The model under review builds one solid part; all positions refer to its coordinate system, in mm. Give positions to 0.01 mm unless a question says otherwise; leave off trailing zeros. Loops run counter-clockwise (first coordinate to the right, second up) from the corner with the lowest first, then second, coordinate; pieces in that order, holes last. Notation, with made-up numbers: M 74.5,6.5 L 124.5,6.5 A9 ccw 124.5,15.5 Z; hole C 85.5,21.25 d8. An arc over 180 degrees is marked long. Put each result on its own line as item: value. Start each with the question number.
from build123d import *

# Parameters (mm, degrees)
F0_W        = 71.12
F0_H        = 140.97
F1_DEPTH    = 15.24
F2_SIZE     = 10.16
F3_SIZE     = 5.08
F4_SIZE     = 5.08
F5_SIZE     = 2.54
F6_SIZE     = 2.54
F7_T1_DEPTH = 24.5183278918
F7_T3_DEPTH = 24.5183278918
F7_T5_DEPTH = 24.5183278918
F7_T7_DEPTH = 24.5183278918


# Not quite as in the source:
# - a fillet or chamfer that OpenCascade refuses, or shapes differently, is made with other operations: its cross-section is extruded or revolved along the edge and cut away or added


with BuildPart() as f1:
    # F0 (on Front) → F1 (new body)
    with BuildSketch(Plane.XZ):
        with Locations((-1.2450981867, 23.9183327848)):
            Rectangle(F0_W, F0_H)
    extrude(amount=F1_DEPTH)

    # F2
    f2_edges = [f1.edges().sort_by_distance(p)[0] for p in [
        (-1.245098, -15.24, 94.403333),
        (34.314902, -15.24, 23.918333),
        (-36.805098, -15.24, 23.918333),
        (-1.245098, -15.24, -46.566667),
    ]]
    chamfer(f2_edges, length=F2_SIZE)

    # F3
    f3_edges = [f1.edges().sort_by_distance(p)[0] for p in [
        (-26.645098, -15.24, 23.918333),
        (-1.245098, -15.24, -36.406667),
        (24.154902, -15.24, 23.918333),
        (-1.245098, -15.24, 84.243333),
    ]]
    chamfer(f3_edges, length=F3_SIZE)

    # F4
    f4_edges = [f1.edges().sort_by_distance(p)[0] for p in [
        (-1.245098, -15.24, 79.163333),
        (-1.245098, -15.24, -31.326667),
        (-21.565098, -15.24, 23.918333),
        (19.074902, -15.24, 23.918333),
    ]]
    chamfer(f4_edges, length=F4_SIZE)

    # F5
    f5_edges = [f1.edges().sort_by_distance(p)[0] for p in [
        (18.881556, -14.267984, 78.969987),
        (-21.371752, -14.267984, 78.969987),
        (-21.371752, -14.267984, -31.133321),
        (18.881556, -14.267984, -31.133321),
    ]]
    chamfer(f5_edges, length=F5_SIZE)

    # F6
    f6_edges = [f1.edges().sort_by_distance(p)[0] for p in [
        (-1.245098, -15.24, 74.083333),
        (-1.245098, -15.24, -26.246667),
    ]]
    chamfer(f6_edges, length=F6_SIZE)

    # F7: chamfer of 2.54 on 4 edges, made by hand

    # F7_s2 → F7_t1 (cut)
    with BuildSketch(Plane(origin=(29.0610725046, 29.0610725046, -29.0610725046), x_dir=(0.7071067812, -0.7071067812, 0), z_dir=(-0.5773502692, -0.5773502692, 0.5773502692))):
        Polygon((25.6566976907, -27.3564258793), (27.8564022163, -23.5464258793), (27.8564022163, -26.0864258793), align=None)
    extrude(amount=F7_T1_DEPTH, mode=Mode.SUBTRACT)

    # F7_s4 → F7_t3 (cut)
    with BuildSketch(Plane(origin=(45.0066276944, 45.0066276944, 45.0066276944), x_dir=(0.7071067812, -0.7071067812, 0), z_dir=(-0.5773502692, -0.5773502692, -0.5773502692))):
        Polygon((27.8564022163, 62.6048997598), (25.6566976907, 66.4148997598), (27.8564022163, 65.1448997598), align=None)
    extrude(amount=F7_T3_DEPTH, mode=Mode.SUBTRACT)

    # F7_s6 → F7_t5 (cut)
    with BuildSketch(Plane(origin=(-45.8366931523, 45.8366931523, 45.8366931523), x_dir=(0.7071067812, 0.7071067812, 0), z_dir=(0.5773502692, -0.5773502692, -0.5773502692))):
        Polygon((-29.6172369585, 61.5882813474), (-27.4175324329, 65.3982813474), (-29.6172369585, 64.1282813474), align=None)
    extrude(amount=F7_T5_DEPTH, mode=Mode.SUBTRACT)

    # F7_s8 → F7_t7 (cut)
    with BuildSketch(Plane(origin=(-29.8911379624, 29.8911379624, -29.8911379624), x_dir=(0.7071067812, 0.7071067812, 0), z_dir=(0.5773502692, -0.5773502692, 0.5773502692))):
        Polygon((-27.4175324329, -26.3398074669), (-29.6172369585, -22.5298074669), (-29.6172369585, -25.0698074669), align=None)
    extrude(amount=F7_T7_DEPTH, mode=Mode.SUBTRACT)


solid = f1.part
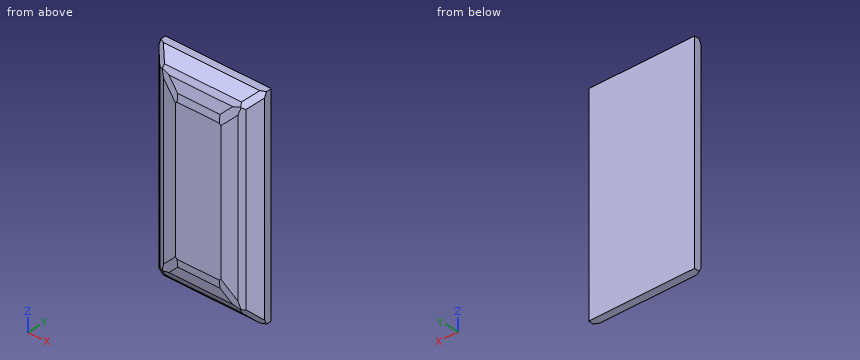
(1) We need section C-C, the plane y = -8.5. Write out the cut boundary in (x, z), plus the area to 3 significant figures.
(2) We need section A-A, the plane z = 8.5. Write out the cut boundary in (x, y).
(3) We need section B-B, the plane x = 5.5. Write out the cut boundary in (y, z).
(4) Insertion check: pin 1 (4 mm diameter, centred on x = 14, y = -8.5, fed in from -Z); pin 2 (1 mm diameter, centred on x = -16.5, y = -11, fed in from +Z); pin 3 (8 mm diameter, centred on y = -10, z = 36.5, fed in from +X). Each pin has a flat end and moves straight along its axis. Give the tip position at first contact, or say it passes through.
(5) We need section D-D, the plane z = 78. Write out the cut boundary in (x, y), plus the area to 3 significant figures.
(6) To check wall thickness, follow L1, parallel to Y at x = 16.5, z = 14; L2, parallel to X at y = -7, z = 20.5; L3, parallel to X at y = -12, z = 79. State the ranges of each line that lie inside material, in increasing order. Write a range as [from, to].
Check sheet entries:
1. outline: M -33.39,-40.04 L -30.27,-43.15 L 27.78,-43.15 L 30.89,-40.04 L 30.89,87.87 L 27.78,90.98 L -30.27,90.98 L -33.39,87.87 Z
1. area: 8,600 mm²
2. outline: M -36.81,-5.08 L -30.24,-11.65 L -26.26,-13.3 L -16.49,-15.24 L 13.99,-15.24 L 23.77,-13.3 L 27.75,-11.65 L 34.31,-5.08 L 34.31,0 L -36.81,0 Z
3. outline: M -15.24,-23.71 L -14.74,-28.74 L -13.3,-36.02 L -11.65,-40 L -5.08,-46.57 L 0,-46.57 L 0,94.4 L -5.08,94.4 L -11.65,87.84 L -13.3,83.86 L -14.74,76.57 L -15.24,71.54 Z
4. pin 1: stops at z = -45.15
4. pin 2: stops at z = 88.98
4. pin 3: stops at x = 33.39
5. outline: M -36.81,-5.08 L -30.24,-11.65 L -26.26,-13.3 L -23.96,-13.75 L -16.84,-14.46 L 14.35,-14.46 L 21.47,-13.75 L 23.77,-13.3 L 27.75,-11.65 L 34.31,-5.08 L 34.31,0 L -36.81,0 Z
5. area: 923 mm²
6. L1: y = [-14.74, 0]
6. L2: x = [-34.89, 32.39]
6. L3: x = [-29.39, 26.9]
